```python
from build123d import *

# Parameters (mm, degrees)
CROQUIS2_W                 = 100
CROQUIS2_H                 = 100
SALIENTE_EXTRUIR1_DEPTH    = 75
CROQUIS3_W                 = 85
CROQUIS3_H                 = 85
CORTAR_EXTRUIR1_DEPTH      = 65
CROQUIS4_W                 = 50
CROQUIS4_H                 = 35
SALIENTE_EXTRUIR2_DEPTH    = 65
CROQUIS5_W                 = 45
CROQUIS5_H                 = 30
CORTAR_EXTRUIR2_DEPTH      = 1
CORTAR_EXTRUIR2_DEPTH_BACK = 65
CROQUIS6_W                 = 15
CROQUIS6_H                 = 10.846969935
CORTAR_EXTRUIR3_DEPTH      = 16
CROQUIS7_W                 = 28.617843409
CROQUIS7_H                 = 7.788560798
CORTAR_EXTRUIR4_DEPTH      = 11
CROQUIS8_W                 = 55.029985219
CROQUIS8_H                 = 51.821882126
SALIENTE_EXTRUIR3_DEPTH    = 75
CROQUIS9_W                 = 51.5
CROQUIS9_H                 = 37.5
CORTAR_EXTRUIR5_DEPTH      = 65
CROQUIS10_R                = 6.5
CORTAR_EXTRUIR6_DEPTH      = 43
CROQUIS11_W                = 5.616805414
CROQUIS11_H                = 14.360656008
SALIENTE_EXTRUIR9_DEPTH    = 3.5
CROQUIS12_W                = 15
CROQUIS12_H                = 15
CORTAR_EXTRUIR7_DEPTH      = 10


with BuildPart() as part:
    # Croquis2 → Saliente-Extruir1 (new body)
    with BuildSketch(Plane(origin=(0, 0, 0), x_dir=(1, 0, 0), z_dir=(0, 1, 0))):
        Rectangle(CROQUIS2_W, CROQUIS2_H)
    extrude(amount=SALIENTE_EXTRUIR1_DEPTH)

    # Croquis3 → Cortar-Extruir1 (cut)
    with BuildSketch(Plane(origin=(0, 75, 0), x_dir=(1, 0, 0), z_dir=(0, 1, 0))):
        Rectangle(CROQUIS3_W, CROQUIS3_H)
    extrude(amount=-CORTAR_EXTRUIR1_DEPTH, mode=Mode.SUBTRACT)

    # Croquis4 → Saliente-Extruir2 (add, through all)
    with BuildSketch(Plane(origin=(0, 10, 0), x_dir=(1, 0, 0), z_dir=(0, 1, 0))):
        with Locations((17.5, -25)):
            Rectangle(CROQUIS4_W, CROQUIS4_H)
    extrude(amount=SALIENTE_EXTRUIR2_DEPTH)

    # Croquis5 → Cortar-Extruir2 (cut, two sides)
    with BuildSketch(Plane(origin=(0, 75, 0), x_dir=(1, 0, 0), z_dir=(0, 1, 0))) as cortar_extruir2_sk:
        with Locations((19.989777708, -27.5)):
            Rectangle(CROQUIS5_W, CROQUIS5_H)
    extrude(amount=CORTAR_EXTRUIR2_DEPTH, mode=Mode.SUBTRACT)
    extrude(cortar_extruir2_sk.sketch, amount=-CORTAR_EXTRUIR2_DEPTH_BACK, mode=Mode.SUBTRACT)

    # Croquis6 → Cortar-Extruir3 (cut)
    with BuildSketch(Plane(origin=(-2.510222292, 0, 0), x_dir=(0, 0, -1), z_dir=(1, 0, 0))):
        with Locations((-35, 15.423484968)):
            Rectangle(CROQUIS6_W, CROQUIS6_H)
    extrude(amount=-CORTAR_EXTRUIR3_DEPTH, mode=Mode.SUBTRACT)

    # Croquis7 → Cortar-Extruir4 (cut)
    with BuildSketch(Plane(origin=(50, 0, 0), x_dir=(0, 0, -1), z_dir=(1, 0, 0))):
        with Locations((14.308921705, 13.894280399)):
            Rectangle(CROQUIS7_W, CROQUIS7_H)
    extrude(amount=-CORTAR_EXTRUIR4_DEPTH, mode=Mode.SUBTRACT)

    # Croquis8 → Saliente-Extruir3 (add, through all)
    with BuildSketch(Plane.XZ):
        with Locations((77.51499261, -24.089058937)):
            Rectangle(CROQUIS8_W, CROQUIS8_H)
    extrude(amount=-SALIENTE_EXTRUIR3_DEPTH)

    # Croquis9 → Cortar-Extruir5 (cut)
    with BuildSketch(Plane(origin=(0, 75, 0), x_dir=(1, 0, 0), z_dir=(0, 1, 0))):
        with Locations((75.75, 23.75)):
            Rectangle(CROQUIS9_W, CROQUIS9_H)
    extrude(amount=-CORTAR_EXTRUIR5_DEPTH, mode=Mode.SUBTRACT)

    # Croquis10 → Cortar-Extruir6 (cut)
    with BuildSketch(Plane(origin=(105.029985219, 0, 0), x_dir=(0, 0, -1), z_dir=(1, 0, 0))):
        with Locations((24.089058937, 24.029815949)):
            Circle(CROQUIS10_R)
    extrude(amount=-CORTAR_EXTRUIR6_DEPTH, mode=Mode.SUBTRACT)

    # Croquis11 → Saliente-Extruir9 (add)
    with BuildSketch(Plane(origin=(105.029985219, 0, 0), x_dir=(0, 0, -1), z_dir=(1, 0, 0))):
        with Locations((17.589058937, 24.029815949)):
            Rectangle(CROQUIS11_W, CROQUIS11_H)
    extrude(amount=-SALIENTE_EXTRUIR9_DEPTH)

    # Croquis12 → Cortar-Extruir7 (cut)
    with BuildSketch(Plane.XY.offset(-42.5)):
        with Locations((-35, 17.5)):
            Rectangle(CROQUIS12_W, CROQUIS12_H)
    extrude(amount=-CORTAR_EXTRUIR7_DEPTH, mode=Mode.SUBTRACT)


solid = part.part
```
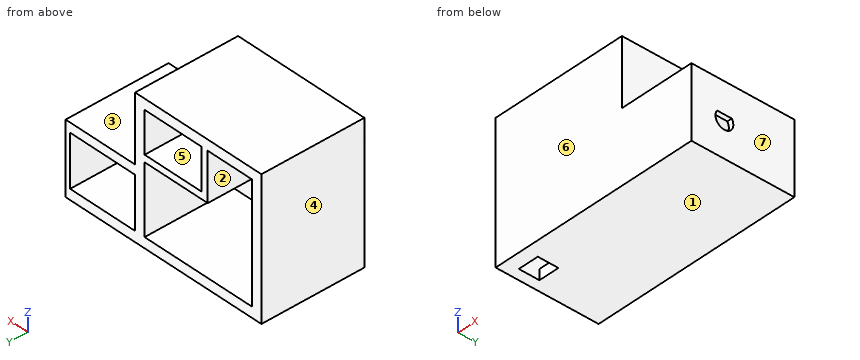
The listing builds one solid part. Answer for the finished solid, in the listing's coordinates (mm). Face numbers are marked on the shaded views. A direction names the side the tool comes from. Round coordinates to 2 decimals unless told otherwise and drop trailing zeros. Loops run counter-clockwise (first coordinate to the right, second up) from the corner with the lowest first, then second, coordinate; pieces in that order, holes last. Notation, with made-up numbers: (-14, 4.25) - (19, 4.25) arc R20 ccw to (19, 17.25) - close; hole circle Ø8 at (0, 34). An arc over 180 degrees is marked (long way). Use one line per item in the form item = value. Start each with the question number.
1. The part is cut by section D-D on x = 25. Determine the outline of the cut face in (y, z).
2. The part is cut by section B-B on x = 46.5. Determine the outline of the cut face in (y, z).
3. Consider line 1 (Z direction, x = -2, y = 12); line 2 (X direction, y = 33.5, z = -18.5); line 3 (X direction, y = 21.5, z = 40.5). Determine where each line is inside the solid, lowest interval first. Write a range as [from, to].
4. A tool of negligible diameter and unlimited length cuts with its end or side. For the marked faces 1, 2 and 3, from which of +Z, -Z, +X, -X, +Y, -Y can it reach the whole face along a straight path? Write none if from no direction.
5. The part is cut by section A-A on z = 29.5. Determine the outline of the cut face in (x, y), then the cut area to 3 significant figures.
6. For a pull along X with two mould halves and no side action, classify the marked faces 4, 5, 6 and 7 as pulls with the +X half, pulls with the -X half, needs draft (parallel to the pull), parting line crosses it, or undercut.
7. The part is cut by section C-C on y = 42.5. Determine the outline of the cut face in (x, z), then the cut area to 3 significant figures.
8. Given pin 1 Ø1.5 at (y, z) = (41, 16) entering from +X, flat-ended and moving along its own axis, determine where the tip first touches the part or whether it passes through.
Geometry check:
q1.outline = (0, -50) - (75, -50) - (75, -42.5) - (10, -42.5) - (10, 7.5) - (75, 7.5) - (75, 12.5) - (10, 12.5) - (10, 42.5) - (75, 42.5) - (75, 50) - (0, 50) - close
q2.outline = (0, -50) - (75, -50) - (75, 50) - (0, 50) - close; hole (10, -28.62) - (17.79, -28.62) - (17.79, 0) - (10, 0) - close
q3.line_1 = [-50, -42.5], [7.5, 12.5], [42.5, 50]
q3.line_2 = [-50, -42.5], [42.5, 50], [101.5, 105.03]
q3.line_3 = [-50, -42.5], [-7.5, -2.51], [42.49, 50]
q4.face_1 = -Z, +X, -X, +Y, -Y
q4.face_2 = +Y
q4.face_3 = +Z, +X, +Y, -Y
q5.outline = (-50, 0) - (50, 0) - (50, 75) - (42.49, 75) - (42.49, 10) - (-42.5, 10) - (-42.5, 75) - (-50, 75) - close; (-7.5, 20.85) - (-2.51, 20.85) - (-2.51, 75) - (-7.5, 75) - close
q5.area = 2,250 mm^2
q6.face_4 = pulls with the -X half
q6.face_5 = undercut
q6.face_6 = needs draft
q6.face_7 = pulls with the +X half
q7.outline = (-50, -50) - (105.03, -50) - (105.03, 1.82) - (50, 1.82) - (50, 50) - (-50, 50) - close; hole (-42.5, -42.5) - (42.5, -42.5) - (42.5, 7.5) - (-7.5, 7.5) - (-7.5, 42.5) - (-42.5, 42.5) - close; hole (-2.51, 12.5) - (42.49, 12.5) - (42.49, 42.5) - (-2.51, 42.5) - close; hole (50, -42.5) - (101.5, -42.5) - (101.5, -5) - (50, -5) - close
q7.area = 4,100 mm^2
q8.pin_1 = 50
